```python
from build123d import *

# Parameters (mm, degrees)
F0_W     = 50.8
F0_H     = 58.169952
F1_DEPTH = 19.558
F2_SIZE  = 5.08
F3_SIZE  = 5.08


with BuildPart() as f1:
    # F0 (on Front) → F1 (new body)
    with BuildSketch(Plane.XZ):
        Rectangle(F0_W, F0_H)
    extrude(amount=F1_DEPTH)

    # F2
    f2_edges = [f1.edges().sort_by_distance(p)[0] for p in [
        (25.4, -9.779, 29.084976),
    ]]
    chamfer(f2_edges, length=F2_SIZE)

    # F3
    f3_edges = [f1.edges().sort_by_distance(p)[0] for p in [
        (25.4, -9.779, -29.084976),
        (-25.4, -19.558, 0),
    ]]
    chamfer(f3_edges, length=F3_SIZE)

    # F4: F1 across face


with BuildPart() as f1_1:
    add(f1.part)
    add(f1.part.mirror(Plane(origin=(-25.4, -7.239, 0), x_dir=(0, -1, 0), z_dir=(-1, 0, 0))))

    # F5: F1 across face


with BuildPart() as f1_2:
    add(f1_1.part)
    add(f1_1.part.mirror(Plane(origin=(-25.4, 0, 0), x_dir=(1, 0, 0), z_dir=(0, 1, 0))))


solid = f1_2.part
```
CAD build for the part. Positions are in the model's coordinates, mm. A direction names the side the tool comes from. Round coordinates to 2 decimals unless told otherwise and drop trailing zeros. Loops run counter-clockwise (first coordinate to the right, second up) from the corner with the lowest first, then second, coordinate; pieces in that order, holes last. Notation, with made-up numbers: M -38.5,67 L -33.5,67 A18 cw -33.5,73 Z; hole C -34.75,-10.75 d2. An arc over 180 degrees is marked long. Use a Markdown table: item, result. Add a question column.
(1) Which spindle directions (+Z, -Z, +X, -X, +Y, -Y) get a long thin tool onto all of the face, cutting with end or side? Do faces 1 (the face through (-22.9, 16.98, -0.41)), 2 (the face through (-53, -19.558, 0)), 3 (the face through (-22.9, -16.98, -0.41)). Say none if no direction does.
(2) Cut at A-A (y = 16). Give the cut face in (x, z), and give its area (3 significant figures).
(3) Drill centre lines: line 1 (X direction, y = 17.5, z = -1); line 2 (X direction, y = 17, z = 16); line 3 (Y direction, x = -26, z = -8.5). Where is each one in solid material? Low to high.
Geometry says:
| question | item | result |
|---|---|---|
| 1 | face 1 | +Z, -Z, +Y |
| 1 | face 2 | +Z, -Z, +X, -X, -Y |
| 1 | face 3 | +Z, -Z, -Y |
| 2 | outline | M -76.2,-24 L -71.12,-29.08 L -26.92,-29.08 L -26.92,29.08 L -71.12,29.08 L -76.2,24 Z; M -23.88,-29.08 L 20.32,-29.08 L 25.4,-24 L 25.4,24 L 20.32,29.08 L -23.88,29.08 Z |
| 2 | area | 5,680 mm² |
| 3 | line 1 | x = -76.2 to -28.42, -22.38 to 25.4 |
| 3 | line 2 | x = -76.2 to -27.92, -22.88 to 25.4 |
| 3 | line 3 | y = -15.08 to 15.08 |
